Check sheet for the modelled part. Datum: model origin and axes. Units: mm. A direction names the side the tool comes from. Give positions to 0.01 mm unless a question says otherwise; leave off trailing zeros. Loops run counter-clockwise (first coordinate to the right, second up) from the corner with the lowest first, then second, coordinate; pieces in that order, holes last.
```python
from build123d import *

# Parameters (mm, degrees)
SALIENTE_EXTRUIR3_DEPTH = 3
CROQUIS4_R              = 10
CROQUIS4_R_2            = 8
CORTAR_EXTRUIR4_DEPTH   = 4


with BuildPart() as part:
    # Croquis3 → Saliente-Extruir3 (new body)
    with BuildSketch(Plane.XY):
        with BuildLine():
            Line((-1.890656386, -4.808889521), (-5.254187971, -8.508437504))
            ThreePointArc((-5.254187971, -8.508437504), (0.814446084, -9.966778696), (6.565812029, -7.54255344))
            Line((6.565812029, -7.54255344), (2.790770571, -4.110385176))
            Line((2.790770571, -4.110385176), (4.808889521, -1.890656386))
            Line((4.808889521, -1.890656386), (8.508437504, -5.254187971))
            ThreePointArc((8.508437504, -5.254187971), (9.966778696, 0.814446084), (7.54255344, 6.565812029))
            Line((7.54255344, 6.565812029), (4.110385176, 2.790770571))
            Line((4.110385176, 2.790770571), (1.890656386, 4.808889521))
            Line((1.890656386, 4.808889521), (5.254187971, 8.508437504))
            ThreePointArc((5.254187971, 8.508437504), (-0.814446084, 9.966778696), (-6.565812029, 7.54255344))
            Line((-6.565812029, 7.54255344), (-2.790770571, 4.110385176))
            Line((-2.790770571, 4.110385176), (-4.808889521, 1.890656386))
            Line((-4.808889521, 1.890656386), (-8.508437504, 5.254187971))
            ThreePointArc((-8.508437504, 5.254187971), (-9.966778696, -0.814446084), (-7.54255344, -6.565812029))
            Line((-7.54255344, -6.565812029), (-4.110385176, -2.790770571))
            Line((-4.110385176, -2.790770571), (-1.890656386, -4.808889521))
        make_face()
    extrude(amount=SALIENTE_EXTRUIR3_DEPTH)

    # Croquis4 → Cortar-Extruir4 (cut, through all)
    with BuildSketch(Plane.XY.offset(3)):
        Circle(CROQUIS4_R)
        Circle(CROQUIS4_R_2, mode=Mode.SUBTRACT)
    extrude(amount=-CORTAR_EXTRUIR4_DEPTH, mode=Mode.SUBTRACT)


solid = part.part
```
(1) Release check for a two-part mould opening along X. For faces 5 (the face through (5.163, 3.948, 1.479)), 6 (the face through (-7.973, -0.655, 1.521)), 7 (the face through (0, 0, 0)), 8 (the face through (-3.8, 3, 1.5)) record: pulls with the +X half, pulls with the -X half, needs draft (parallel to the pull), parting line crosses it, or undercut.
(2) Section check C-C on z = 0.55. Record the boundary of the cut face in (x, y), plus the area to 3 significant figures.
(3) Section check B-B on y = -4.5. Record the boundary of the cut face in (x, z).
(4) Section check D-D on x = -6.75. Record the boundary of the cut face in (y, z), plus the area to 3 significant figures.
(5) Access from +Z, -Z, +X, -X, +Y, -Y to the whole of each face (thin tool, end or side, straight path). Record for faces 1 (the face through (-5.163, -3.948, 1.479)), 2 (the face through (-3, -3.8, 1.5)), 3 (the face through (-3.948, 5.163, 1.479)), 4 (the face through (3.948, -5.163, 1.479)).
(6) Material ranges on line 1 (Y direction, x = -3.75, z = 1.65); line 2 (X direction, y = 3.5, z = 1.65); line 3 (X direction, y = -3.25, z = 1.25), recorded low to high.
(7) Section check A-A on x = -3.5. Record the boundary of the cut face in (y, z), plus the area to 3 significant figures.
Computed values:
1. face 5: undercut
1. face 6: pulls with the -X half
1. face 7: needs draft
1. face 8: undercut
2. outline: (-7, 3.88) arc R8 ccw to (-6.19, -5.07) - (-4.11, -2.79) - (-1.89, -4.81) - (-3.88, -7) arc R8 ccw to (5.07, -6.19) - (2.79, -4.11) - (4.81, -1.89) - (7, -3.88) arc R8 ccw to (6.19, 5.07) - (4.11, 2.79) - (1.89, 4.81) - (3.88, 7) arc R8 ccw to (-5.07, 6.19) - (-2.79, 4.11) - (-4.81, 1.89) - close
2. area: 164 mm2
3. outline: (-6.61, 0) - (-5.66, 0) - (-5.66, 3) - (-6.61, 3) - close; (-2.23, 0) - (3.22, 0) - (3.22, 3) - (-2.23, 3) - close
4. outline: (-4.29, 0) - (3.66, 0) - (3.66, 3) - (-4.29, 3) - close
4. area: 23.8 mm2
5. face 1: +Z, -Z, -Y
5. face 2: +Z, -Z
5. face 3: +Z, -Z, -X
5. face 4: +Z, -Z, +X
6. line 1: y = -7.07 to -6.85, -3.12 to 3.06, 4.98 to 7.07
6. line 2: x = -7.19 to -6.58, -3.35 to 3.33, 4.76 to 7.19
6. line 3: x = -7.31 to -4.53, -3.61 to 3.57, 6.3 to 7.31
7. outline: (-7.19, 0) - (-6.58, 0) - (-6.58, 3) - (-7.19, 3) - close; (-3.35, 0) - (3.33, 0) - (3.33, 3) - (-3.35, 3) - close; (4.76, 0) - (7.19, 0) - (7.19, 3) - (4.76, 3) - close
7. area: 29.2 mm2
